The listing builds one solid part. Answer for the finished solid, in the listing's coordinates (mm). A direction names the side the tool comes from. Coordinates: 2 decimals unless noted, no trailing zeros. Loops run counter-clockwise (first coordinate to the right, second up) from the corner with the lowest first, then second, coordinate; pieces in that order, holes last. Notation, with made-up numbers: (34.25, -20.5) - (46.25, -20.5) arc R12 ccw to (46.25, -1.5) - close; hole circle Ø7 at (11, 68.25). An arc over 180 degrees is marked (long way). Put each result on its own line as item: value.
```python
from build123d import *

# Parameters (mm, degrees)
SKETCH1_W           = 16
SKETCH1_H           = 16
BOSS_EXTRUDE1_DEPTH = 7
SKETCH2_W           = 12
SKETCH2_H           = 12
CUT_EXTRUDE1_DEPTH  = 6
SKETCH3_R           = 1.25
BOSS_EXTRUDE2_DEPTH = 2
FILLET1_R           = 1
SKETCH4_R           = 0.5
BOSS_EXTRUDE3_DEPTH = 2


with BuildPart() as part:
    # Sketch1 → Boss-Extrude1 (new body)
    with BuildSketch(Plane(origin=(0, 0, 0), x_dir=(1, 0, 0), z_dir=(0, 1, 0))):
        Rectangle(SKETCH1_W, SKETCH1_H)
    extrude(amount=BOSS_EXTRUDE1_DEPTH)

    # Sketch2 → Cut-Extrude1 (cut)
    with BuildSketch(Plane(origin=(0, 7, 0), x_dir=(1, 0, 0), z_dir=(0, 1, 0))):
        Rectangle(SKETCH2_W, SKETCH2_H)
    extrude(amount=-CUT_EXTRUDE1_DEPTH, mode=Mode.SUBTRACT)

    # Sketch3 → Boss-Extrude2 (add)
    with BuildSketch(Plane(origin=(0, 1, 0), x_dir=(1, 0, 0), z_dir=(0, 1, 0))):
        Circle(SKETCH3_R)
    extrude(amount=BOSS_EXTRUDE2_DEPTH)

    # Fillet1
    fillet1_edges = [part.edges().sort_by_distance(p)[0] for p in [
        (-1.25, 3, 0),
    ]]
    fillet(fillet1_edges, radius=FILLET1_R)

    # Sketch4 → Boss-Extrude3 (add)
    with BuildSketch(Plane(origin=(0, 7, 0), x_dir=(1, 0, 0), z_dir=(0, 1, 0))):
        with Locations((-7, 7)):
            Circle(SKETCH4_R)
        with Locations((7, 7)):
            Circle(SKETCH4_R)
        with Locations((7, -7)):
            Circle(SKETCH4_R)
        with Locations((-7, -7)):
            Circle(SKETCH4_R)
    extrude(amount=BOSS_EXTRUDE3_DEPTH)


solid = part.part
```
1) Each of these flat-tipped pins is pushed along its axis until it touches: pin 1 (0.6 mm diameter, centred on x = 0, z = 0, fed in from +Y); pin 2 (5 mm diameter, centred on y = 7.5, z = -5.5, fed in from -X); pin 3 (3.5 mm diameter, centred on x = -2.5, z = 0, fed in from +Y); pin 4 (1 mm diameter, centred on x = 2.5, z = -4.5, fed in from +Y). Where does it stop, or does it pass through?
Found:
pin 1: stops at y = 3
pin 2: stops at x = -8
pin 3: stops at y = 2.87
pin 4: stops at y = 1
2) The part is cut by section A-A (y = 1.25). Give the vertices of the cut face in (x, z).
Found:
outline: (-8, -8) - (8, -8) - (8, 8) - (-8, 8) - close; circle Ø2.5 at (0, 0); hole (-6, -6) - (6, -6) - (6, 6) - (-6, 6) - close
3) For a pull along X with two mould halves and no side action, classify faces 3 (the face through (-6.769, 7.986, 7.444)), 4 (the face through (8, 3, 0)), 5 (the face through (6, 4, 0)), 6 (the face through (0, 0, 0)) as pulls with the +X half, pulls with the -X half, needs draft (parallel to the pull), parting line crosses it, or undercut.
Found:
face 3: undercut
face 4: pulls with the +X half
face 5: undercut
face 6: needs draft
4) The part is cut by section D-D (z = 7). Give the vertices of the cut face in (x, y).
Found:
outline: (-8, 0) - (8, 0) - (8, 7) - (7.5, 7) - (7.5, 9) - (6.5, 9) - (6.5, 7) - (-6.5, 7) - (-6.5, 9) - (-7.5, 9) - (-7.5, 7) - (-8, 7) - close
5) For faces 1 (the face through (0, 3, 8)), 2 (the face through (-6, 4, 0)), determine the directions among +Z, -Z, +X, -X, +Y, -Y from which every point of the face is accessible in a straight line to the end or side of a thin tool.
Found:
face 1: +Z, +X, -X, +Y, -Y
face 2: +Y
6) Straight lines are drawn through the part: L1, parallel to X at y = 3.75, z = -3.5; L2, parallel to X at y = 1.25, z = -1. For each, find the intervals that lie inside material, in ascending order. Write a range as [from, to].
Found:
L1: x = [-8, -6], [6, 8]
L2: x = [-8, -6], [-0.75, 0.75], [6, 8]
7) The part is cut by section B-B (x = 2). Give the vertices of the cut face in (y, z), and give its area (3 significant figures).
Found:
outline: (0, -8) - (7, -8) - (7, -6) - (1, -6) - (1, 6) - (7, 6) - (7, 8) - (0, 8) - close
area: 40.0 mm^2
8) The part is cut by section C-C (y = 4). Give the vertices of the cut face in (x, z), and give its area (3 significant figures).
Found:
outline: (-8, -8) - (8, -8) - (8, 8) - (-8, 8) - close; hole (-6, -6) - (6, -6) - (6, 6) - (-6, 6) - close
area: 112 mm^2
